Input: dimensioned drawing with shaded views. Units: mm. Origin: part minimum x, y, z. A direction names the side the tool comes from. Coordinates: 2 decimals unless noted, no trailing zeros. Order: outer loops, then holes, each group sorted by start corner. A loop starts at its lowest first (then second) coordinate and runs counter-clockwise, first axis right, second up. Notation, with made-up numbers: (24.5, 57) -> (45.5, 57) arc R11 cw to (45.5, 75) -> close; hole circle Ø7 at (73.25, 68.25). An arc over 180 degrees is marked (long way). Answer in a Markdown table with one row per item. Add a question column.
1) Ray query, line 1 (X direction, y = 77, z = 20); line 2 (Z direction, x = 124, y = 51.5); line 3 (Y direction, x = 237.5, z = 81). Return the intervals inside material, ascending. Write a range as from..to.
2) Section query A-A on z = 118. Return the cut outline in (x, y), then the cut area to 3 significant figures.
3) Section query C-C on y = 75. Return the cut outline in (x, z), then the cut area to 3 significant figures.
4) Section query B-B on x = 251.5. Return the cut outline in (y, z).
5) Contact query for flat-ended pins moving along their axis: P1, Ø12, axis at x = 203.5, z = 106, coming from the +Y side; P2, Ø1.5, axis at x = 101, z = 82.5, coming from the -Y side; P3, Ø5, axis at x = 223.5, y = 71, coming from the +Z side. Output: stop coordinate, or through.
6) Set-up query: the marked faces 1, 2, 3, 4 and 5. Return all of +Z, -Z, +X, -X, +Y, -Y with unobstructed straight access to the full face (end or side cutting, diameter ignored); none if empty.
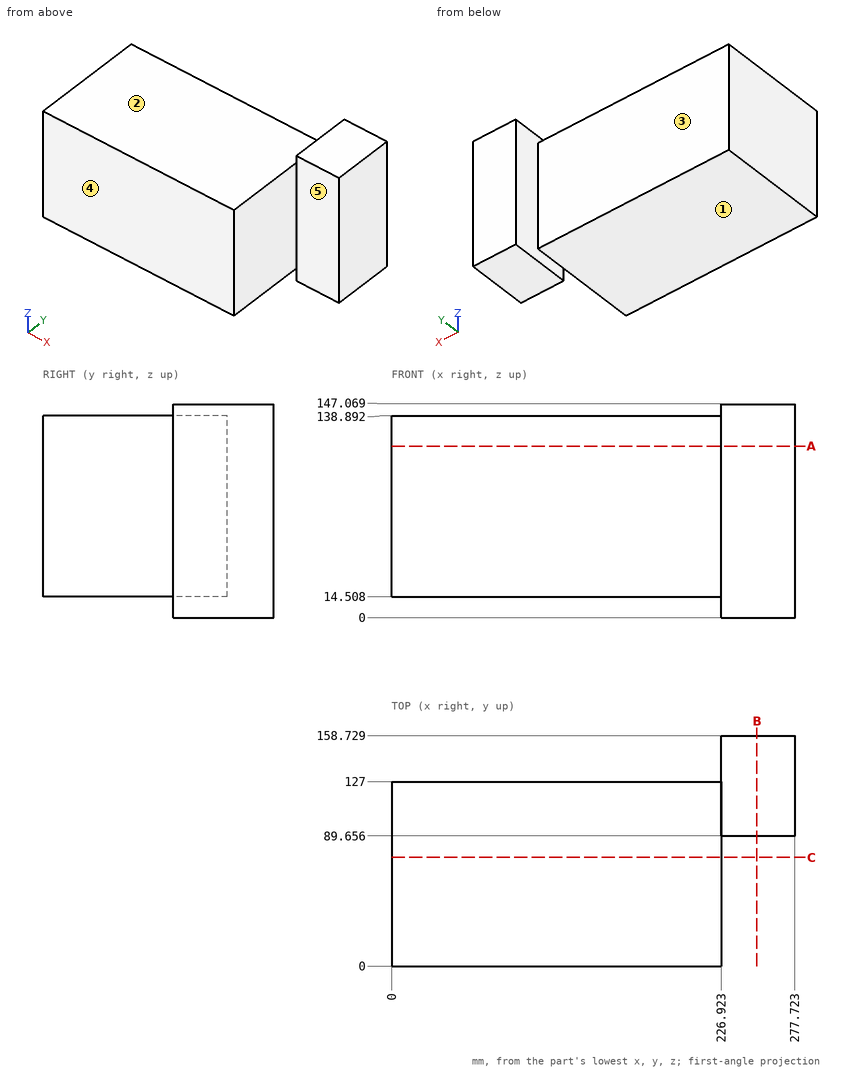
Result:
| question | item | result |
|---|---|---|
| 1 | line 1 | 0..226.92 |
| 1 | line 2 | 14.51..138.89 |
| 1 | line 3 | 89.66..158.73 |
| 2 | outline | (0, 0) -> (226.92, 0) -> (226.92, 89.66) -> (277.72, 89.66) -> (277.72, 158.73) -> (226.92, 158.73) -> (226.92, 127) -> (0, 127) -> close |
| 2 | area | 32,300 mm2 |
| 3 | outline | (0, 14.51) -> (226.92, 14.51) -> (226.92, 138.89) -> (0, 138.89) -> close |
| 3 | area | 28,200 mm2 |
| 4 | outline | (89.66, 0) -> (158.73, 0) -> (158.73, 147.07) -> (89.66, 147.07) -> close |
| 5 | P1 | y = 127 |
| 5 | P2 | y = 0 |
| 5 | P3 | z = 138.89 |
| 6 | face 1 | -Z, -X, +Y, -Y |
| 6 | face 2 | +Z, -X, +Y, -Y |
| 6 | face 3 | +Z, -Z, -X, +Y |
| 6 | face 4 | +Z, -Z, +X, -X, -Y |
| 6 | face 5 | +Z, -Z, +X, -Y |
